Autodesk Inventor part; units mm, degrees
ref_plane "YZ Plane" through (0, 0, 0) normal (1, 0, 0) x (0, 1, 0)
ref_plane "XZ Plane" through (0, 0, 0) normal (0, 1, 0) x (-1, 0, 0)
ref_plane "XY Plane" through (0, 0, 0) normal (0, 0, 1) x (1, 0, 0)
sketch "Sketch1" plane through (0, 0, 0) normal (0, 1, 0) x (-1, 0, 0)
  line L0 (47.4221, 0) -> (47.4221, -5)
  line L1 (47.4221, -5) -> (45.5221, -5)
  line L2 (45.5221, -5) -> (45.5221, 1)
  line L3 (47.4221, 0) -> (52.4221, 0)
  line L4 (52.4221, 0) -> (52.4221, -12)
  line L5 (52.4221, -12) -> (29.5221, -12)
  line L6 (45.5221, 1) -> (40.5221, 1)
  line L7 (29.5221, -12) -> (29.5221, 8)
  line L8 (29.5221, 8) -> (40.5221, 8)
  line L9 (40.5221, 8) -> (40.5221, 1)
  line L10 (47.4221, -5) -> (52.4221, -5)
  line L11 (52.4221, -5) -> (52.4221, -16)
  line L12 (52.4221, -16) -> (29.5221, -16)
  line L13 (29.5221, -16) -> (29.5221, -12)
  point P0 (0, 0)
  dimension "d0" = 5
  dimension "d1" = 1.9
  dimension "d2" = 6
  dimension "d4" = 5
  dimension "d5" = 12
  dimension "d6" = 5
  dimension "d7" = 20
  dimension "d8" = 11
  dimension "d9" = 7
  dimension "d10" = 11
extrude "Extrusion1" add sketch "Sketch1" along normal blind 100
sketch "Sketch2" plane through (-52.4221, 0, -16) normal (-1, 0, 0) x (0, 0, 1)
  line L0 (0, 0) -> (0, 100)
  line L1 (0, 0) -> (5, 0)
  line L2 (24, 0) -> (0, 0)
  line L3 (5, 0) -> (5, 5)
  circle A0 centre (5, 5) radius 1.5
  line L4 (0, 100) -> (5, 100)
  line L5 (24, 100) -> (0, 100)
  line L6 (5, 100) -> (5, 95)
  circle A1 centre (5, 95) radius 1.5
  point P0 (16, 0)
  dimension "d13" = 5
  dimension "d14" = 5
  dimension "d15" = 3
  dimension "d16" = 5
  dimension "d17" = 5
  dimension "d18" = 3
hole "Hole1" at (-52.4221, 5, -11) at (-52.4221, 95, -11) direction (1, 0, 0) diameter 3 end through all
fillet "Fillet1" radius 2 12 edges at (-52.4221, 50, -16) (-52.4221, 0, -8) (-52.4221, 100, -8) (-40.9721, 100, -16) (-40.9721, 0, -16) (-40.5221, 50, 8) (-40.5221, 0, 4.5) (-43.0221, 0, 1) (-49.9221, 0, 0) (-49.9221, 100, 0) (-43.0221, 100, 1) (-40.5221, 100, 4.5)
properties part number "Wal Mount"
Build history of the part. All positions in model axes, mm. A direction names the side the tool comes from. Round coordinates to 2 decimals unless told otherwise and drop trailing zeros. Order: outer loops, then holes, each group sorted by start corner. A loop starts at its lowest first (then second) coordinate and runs counter-clockwise, first axis right, second up. Notation, with made-up numbers: M 15.25,66.25 L 37.25,66.25 A20 ccw 37.25,84.25 Z; hole C 48.5,-38.5 d2. An arc over 180 degrees is marked long. Use CSV: the item, a comma, the result in double quotes. Start each with the question number.
(1) Cut at B-B on z = -11. List the corners of the cut face in (x, y), then the cut area to 3 significant figures.
(2) Cut at C-C on y = 43. List the corners of the cut face in (x, z).
(3) Drill centre lines: probe 1 along Y at (x, z) = (-43.25, -11); probe 2 along X at (y, z) = (66.5, -2.5); probe 3 along Z at (x, y) = (-43.5, 5). Where is each one in solid material? Low to high.
(4) Cut at A-A on y = 5. List the corners of the cut face in (x, z), then the cut area to 3 significant figures.
(5) Flat gauge pins, fed straight in: P1, Ø1, axis at x = -32, z = 4.5, coming from the -Y side; P2, Ø1.5, axis at x = -49.5, y = 61.5, coming from the +Z side; P3, Ø1.5, axis at y = 62.5, z = 4.5, coming from the -X side; P4, Ø1.5, axis at x = -42, y = 54, coming from the +Z side. Where does each tip first touch, or does it go through?
(6) Mould opens along X. For faces 5 (the face through (-29.522, 49, -4)), 6 (the face through (-47.422, 49, -2)), 7 (the face through (-39.92, 0.57, 3.44)), 8 (the face through (-39.83, 0.57, -15.4)) say: +X half, -X half, draft (parallel to the pull), parting line (faces both ways), or undercut.
(7) Tool access for faces 1 (the face through (-42.75, 0.6, 0.43)), 2 (the face through (-50, 49, 0)), 3 (the face through (-34, 49, 8)), 4 (the face through (-49.4, 99.4, -0.57)): list every direction of +Z, -Z, +X, -X, +Y, -Y with a clear straight run to the whole face (end or side of a thin tool).
Findings:
1,outline,"M -52.42,2 A2 ccw -50.42,0 L -29.52,0 L -29.52,3.5 L -52.42,3.5 Z; M -52.42,6.5 L -29.52,6.5 L -29.52,93.5 L -52.42,93.5 Z; M -52.42,96.5 L -29.52,96.5 L -29.52,100 L -50.42,100 A2 ccw -52.42,98 Z"
1,area,"2,150 mm^2"
2,outline,"M -52.42,-14 A2 ccw -50.42,-16 L -29.52,-16 L -29.52,8 L -38.52,8 A2 ccw -40.52,6 L -40.52,1 L -45.52,1 L -45.52,-5 L -47.42,-5 L -47.42,0 L -52.42,0 Z"
3,probe 1,"y = 0 to 3.5, 6.5 to 93.5, 96.5 to 100"
3,probe 2,"x = -52.42 to -47.42, -45.52 to -29.52"
3,probe 3,"z = -16 to -12.5, -9.5 to 1"
4,outline,"M -52.42,-14 A2 ccw -50.42,-16 L -29.52,-16 L -29.52,-12.5 L -52.42,-12.5 Z; M -52.42,-9.5 L -29.52,-9.5 L -29.52,8 L -38.52,8 A2 ccw -40.52,6 L -40.52,1 L -45.52,1 L -45.52,-5 L -47.42,-5 L -47.42,0 L -52.42,0 Z"
4,area,"379 mm^2"
5,P1,"stops at y = 0"
5,P2,"stops at z = 0"
5,P3,"stops at x = -40.52"
5,P4,"stops at z = 1"
6,face 5,"+X half"
6,face 6,"undercut"
6,face 7,"-X half"
6,face 8,"draft"
7,face 1,"+Z, -X, -Y"
7,face 2,"+Z, -X, +Y, -Y"
7,face 3,"+Z, +X, -X, +Y, -Y"
7,face 4,"+Z, -X, +Y"
